Answer from the drawing. Dimensions are ordinates in mm from the lowest x, y and z of the part. A direction names the side the tool comes from. Round coordinates to 2 decimals unless told otherwise and drop trailing zeros. Loops run counter-clockwise (first coordinate to the right, second up) from the corner with the lowest first, then second, coordinate; pieces in that order, holes last. Notation, with made-up numbers: (38.25, 40) - (52.25, 40) arc R21 cw to (52.25, 77) - close; hole circle Ø10 at (11.25, 53). An arc over 180 degrees is marked (long way). Use CSV: the item, a comma, the result in double quotes. Start each with the question number.
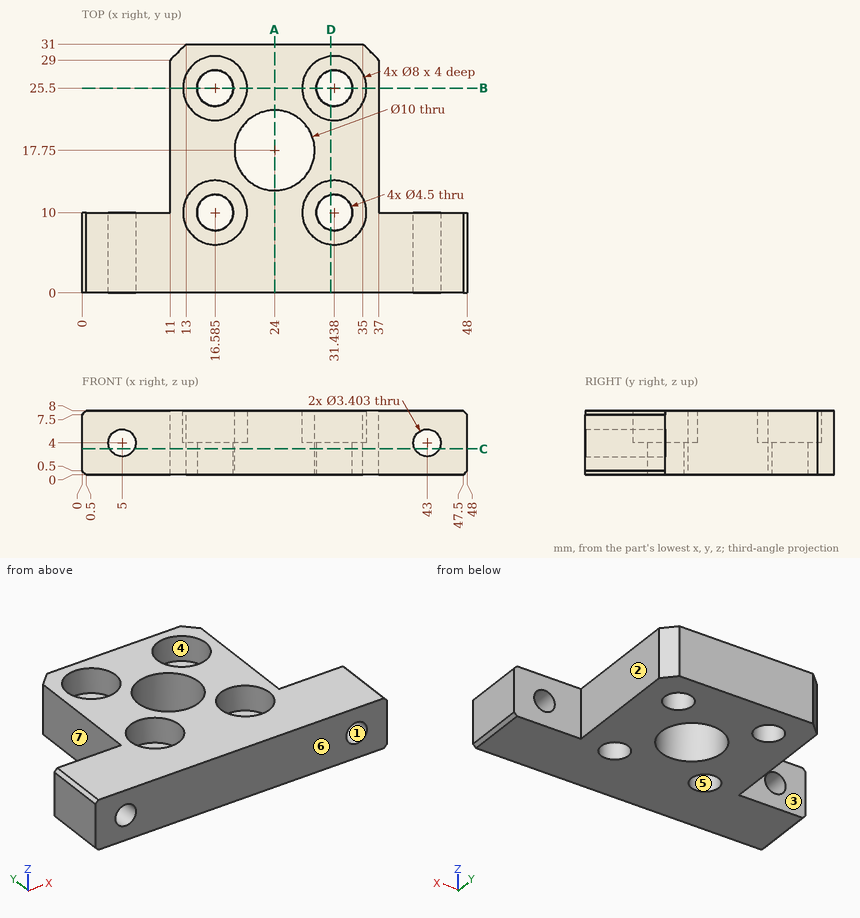
Item 1: A cutting plane is placed at B-B (y = 25.5). Determine the outline of the cut face in (x, z) (1 decimal).
Item 2: A cutting plane is placed at D-D (x = 31). Determine the outline of the cut face in (y, z), plus the area to 3 significant figures.
Item 3: Each of these flat-tipped pins is pushed along its axis until it touches: pin 1 Ø4 at (x, z) = (37.5, 2.5) entering from +Y; pin 2 Ø5 at (x, y) = (31.44, 25.5) entering from +Z. Where does it stop, or does it pass through?
Item 4: A cutting plane is placed at A-A (x = 24). Determine the outline of the cut face in (y, z), plus the area to 3 significant figures.
Item 5: Which of the six approach directions +Z, -Z, +X, -X, +Y, -Y give full straight-line access (tool end or side, diameter ignored) to the marked faces 1, 2, 3 and 4?
Item 6: Find the intervals of material crossed by probe 1 along X at (y, z) = (25.5, 1.7) (1 decimal); probe 2 along Y at (x, z) = (24, 3.5); probe 3 along X at (y, z) = (7, 3.75), in increasing order. Write a range as [from, to].
Item 7: A cutting plane is placed at C-C (z = 3.25). State how many separate pieces and enclosed holes the cut face has, plus the area to 3 significant figures.
Item 8: The mould has two halves that part along Y. Classify the marked faces 5, 6 and 7: pulls with the +Y half, pulls with the -Y half, needs draft (parallel to the pull), parting line crosses it, or undercut.
Result sheet:
1,outline,"(11, 0) - (14.3, 0) - (14.3, 4) - (12.6, 4) - (12.6, 8) - (11, 8) - close; (18.8, 0) - (29.2, 0) - (29.2, 4) - (27.4, 4) - (27.4, 8) - (20.6, 8) - (20.6, 4) - (18.8, 4) - close; (33.7, 0) - (37, 0) - (37, 8) - (35.4, 8) - (35.4, 4) - (33.7, 4) - close"
2,outline,"(0, 0) - (7.79, 0) - (7.79, 4) - (6.02, 4) - (6.02, 8) - (0, 8) - close; (12.21, 0) - (23.29, 0) - (23.29, 4) - (21.52, 4) - (21.52, 8) - (13.98, 8) - (13.98, 4) - (12.21, 4) - close; (27.71, 0) - (31, 0) - (31, 8) - (29.48, 8) - (29.48, 4) - (27.71, 4) - close"
2,area,"149 mm^2"
3,pin 1,"y = 30.5"
3,pin 2,"z = 4"
4,outline,"(0, 0) - (12.75, 0) - (12.75, 8) - (0, 8) - close; (22.75, 0) - (31, 0) - (31, 8) - (22.75, 8) - close"
4,area,"168 mm^2"
5,face 1,"+Y, -Y"
5,face 2,"+Z, -Z, +X, +Y"
5,face 3,"+Z, -Z, -X, +Y"
5,face 4,"+Z"
6,probe 1,"[11, 14.3], [18.8, 29.2], [33.7, 37]"
6,probe 2,"[0, 12.75], [22.75, 31]"
6,probe 3,"[0, 3.32], [6.68, 41.32], [44.68, 48]"
7,separate pieces,"3"
7,enclosed holes,"5"
7,area,"819 mm^2"
8,face 5,"undercut"
8,face 6,"pulls with the -Y half"
8,face 7,"needs draft"
